Can you work these out from the model? Positions are in its coordinate system, mm. A direction names the side the tool comes from. Give positions to 0.01 mm unless a question says otherwise; leave off trailing zeros. Order: outer loops, then holes, each group sorted by start corner. A loop starts at its lowest first (then second) coordinate and runs counter-clockwise, first axis right, second up.
Item 1: If I drill on line 1 along X through (y, z) = (-21.55, 0); line 2 along X through (y, z) = (-23.2, 0); line 3 along X through (y, z) = (-21.65, 2.75), over which ranges is the centre line in solid material (lowest first)?
Item 2: I want a section at C-C, the plane z = -5.75. Write out the boundary of the cut face in (x, y), then the cut area to 3 significant figures.
Item 3: I want a section at A-A, the plane y = -21.15. Write out the boundary of the cut face in (x, z), then the cut area to 3 significant figures.
Item 4: Which directions (+Z, -Z, +X, -X, +Y, -Y) give clear straight access to the entire face, cutting with the end or side of a thin tool? Please do faces 5 (the cylindrical face through (-10.64, -21.87, 4.49)), 6 (the flat face through (-10.4, -22.03, -5.37)), 7 (the flat face through (-3, -23.5, -4)).
Item 5: I'm going to push flat-ended pins straight in: pin 1 Ø1.2 at (y, z) = (-22.5, 3) entering from +X; pin 2 Ø0.8 at (x, y) = (-1.5, -22.5) entering from -Z; pin 3 Ø6.5 at (x, z) = (1, 0) entering from +Y. Where does each tip first touch, or does it pass through?
Item 6: If we mould it in two halves opening along X, with no side actions, what happens to faces 1 (the flat face through (-2.724, -23.245, 0.537)), 2 (the cylindrical face through (-8.025, -22.028, 7.208)), 3 (the flat face through (4, -22, -4)), 4 (the flat face through (-7, -20, 7))? For each: +X half, -X half, draft (parallel to the pull), parting line (faces both ways), or undercut.
Item 7: I want a section at B-B, the plane x = 13. Write out the boundary of the cut face in (y, z).
Item 8: I want a section at D-D, the plane x = 2. Write out the boundary of the cut face in (y, z), then the cut area to 3 significant figures.
```python
from build123d import *

# Parameters (mm, degrees)
PAD096_DEPTH    = 4
SKETCH294_R     = 1.5
POCKET172_DEPTH = 6
SKETCH295_R     = 0.95
POCKET173_DEPTH = 1.5
SKETCH299_W     = 4.5
SKETCH299_H     = 8
POCKET175_DEPTH = 3
POCKET176_DEPTH = 5
POCKET177_DEPTH = 5
PAD107_DEPTH    = 2.5


with BuildPart() as part:
    # Sketch278 → Pad096 (new body)
    with BuildSketch(Plane.XZ.offset(24)):
        with BuildLine():
            Line((-17, -2.25), (-17, 2.25))
            ThreePointArc((-7, 7.25), (-12.5901699437, 5.9303398875), (-17, 2.25))
            Line((-7, 7.25), (0, 7.25))
            Line((0, 7.25), (0, -9.3))
            ThreePointArc((-3.9748544782, -8.4077661645), (-2.0368817676, -9.0742003871), (0, -9.3))
            Line((-3.9748544782, -8.4077661645), (-17, -2.25))
        make_face()
    pad096 = extrude(amount=-PAD096_DEPTH)

    # Sketch294 (on Face8 of Pad096) → Pocket172 (cut)
    with BuildSketch(Plane(origin=(0, -20, 0), x_dir=(1, 0, 0), z_dir=(0, 1, 0))):
        with Locations((-13, 0)):
            Circle(SKETCH294_R)
    pocket172 = extrude(amount=-POCKET172_DEPTH, mode=Mode.SUBTRACT)

    # Sketch295 (on Face5 of Pocket172) → Pocket173 (cut)
    with BuildSketch(Plane(origin=(0, -20, 0), x_dir=(1, 0, 0), z_dir=(0, 1, 0))):
        with BuildLine():
            Line((0, 9), (0, -9))
            ThreePointArc((-7.5, -4.9749371855), (-4.2559114964, -7.9301461106), (0, -9))
            Line((-7.5, -4.9749371855), (-7.5, 4.9749371855))
            ThreePointArc((0, 9), (-4.2559114964, 7.9301461106), (-7.5, 4.9749371855))
        make_face()
        with Locations((-6, 0)):
            Circle(SKETCH295_R, mode=Mode.SUBTRACT)
    pocket173 = extrude(amount=-POCKET173_DEPTH, mode=Mode.SUBTRACT)

    # Sketch299 (on Face5 of Pocket172) → Pocket175 (cut)
    with BuildSketch(Plane(origin=(0, -20, 0), x_dir=(1, 0, 0), z_dir=(0, 1, 0))):
        with Locations((-2.25, 0)):
            Rectangle(SKETCH299_W, SKETCH299_H)
    pocket175 = extrude(amount=-POCKET175_DEPTH, mode=Mode.SUBTRACT)

    # Mirrored012: Pad096, Pocket172, Pocket173, Pocket175 across Sketch278 V_Axis
    add(pad096.mirror(Plane(origin=(0, -24, 0), x_dir=(0, -1, 0), z_dir=(1, 0, 0))))
    add(pocket172.mirror(Plane(origin=(0, -24, 0), x_dir=(0, -1, 0), z_dir=(1, 0, 0))), mode=Mode.SUBTRACT)
    add(pocket173.mirror(Plane(origin=(0, -24, 0), x_dir=(0, -1, 0), z_dir=(1, 0, 0))), mode=Mode.SUBTRACT)
    add(pocket175.mirror(Plane(origin=(0, -24, 0), x_dir=(0, -1, 0), z_dir=(1, 0, 0))), mode=Mode.SUBTRACT)

    # Sketch300 → Pocket176 (cut)
    with BuildSketch(Plane.XZ.offset(24)):
        Polygon((-9, 0), (-13.5886114908, 6.5532163543), (-10.3120033137, 8.8475220997), (-5.7233918228, 2.2943057454), align=None)
    extrude(amount=-POCKET176_DEPTH, mode=Mode.SUBTRACT)

    # Sketch301 → Pocket177 (cut)
    with BuildSketch(Plane.XZ.offset(23.5)):
        with BuildLine():
            ThreePointArc((-3.5, -7.7459666924), (0, -8.5), (3.5, -7.7459666924))
            Line((3.5, -7.7459666924), (3.5, -3.7459666924))
            Line((3.5, -3.7459666924), (-6.7056942546, 3.2766081772))
            Line((-6.7056942546, 3.2766081772), (-9, 0))
            Line((-9, 0), (-3.5, -7.7459666924))
        make_face()
    extrude(amount=-POCKET177_DEPTH, mode=Mode.SUBTRACT)

    # Sketch302 (on Face13 of Pocket177) → Pad107 (join)
    with BuildSketch(Plane(origin=(-6.039090645, 0, -4.2286167935), x_dir=(-0.5735764364, 0, 0.8191520443), z_dir=(0.8191520443, 0, 0.5735764364))):
        with BuildLine():
            Line((12, 20), (12, 23))
            ThreePointArc((7.4, 21.5), (9.8191940807, 21.8844714859), (12, 23))
            Line((7.4, 21.5), (7.4, 20))
            Line((7.4, 20), (12, 20))
        make_face()
    extrude(amount=PAD107_DEPTH)


solid = part.part
```
Results list:
1. line 1: x = -17 to -14.5, -11.5 to -9, 4.5 to 11.5, 14.5 to 17
1. line 2: x = -17 to -14.5, -11.5 to -9, -1.94 to 11.5, 14.5 to 17
1. line 3: x = -16.6 to -10.93, -5.94 to -4.5, 4.5 to 16.6
2. outline: (-9.6, -24) - (9.6, -24) - (9.6, -20) - (6.92, -20) - (6.92, -21.5) - (3.5, -21.5) - (3.5, -23.5) - (-4.92, -23.5) - (-4.92, -21.5) - (-6.92, -21.5) - (-6.92, -20) - (-9.6, -20) - close
2. area: 39.2 mm2
3. outline: (-17, -2.25) - (-3.97, -8.41) arc R9.3 ccw to (3.97, -8.41) - (17, -2.25) - (17, 2.25) arc R12.5 ccw to (7, 7.25) - (5.33, 7.25) arc R9 cw to (7.5, 4.97) - (7.5, -4.97) arc R9 cw to (-7.5, -4.97) - (-7.5, -2.11) - (-9, 0) - (-10.28, 1.83) - (-8.24, 3.27) - (-10.87, 7.04) - (-12.92, 5.6) - (-13, 5.71) arc R12.5 ccw to (-17, 2.25) - close; (-9.07, 7.08) - (-7.5, 4.83) - (-7.5, 4.97) arc R9 cw to (-5.33, 7.25) - (-7, 7.25) arc R12.5 ccw to start; circle Ø1.9 at (6, 0); hole circle Ø3 at (-13, 0); hole circle Ø3 at (13, 0)
3. area: 180 mm2
4. face 5: -Y
4. face 6: -Z, -X, +Y, -Y
4. face 7: +Y
5. pin 1: stops at x = 16.89
5. pin 2: stops at z = -9.23
5. pin 3: stops at y = -23
6. face 1: undercut
6. face 2: -X half
6. face 3: undercut
6. face 4: draft
7. outline: (-24, -4.14) - (-20, -4.14) - (-20, -1.5) - (-24, -1.5) - close; (-24, 1.5) - (-20, 1.5) - (-20, 5.72) - (-24, 5.72) - close
8. outline: (-24, -9.08) - (-20, -9.08) - (-20, -8.77) - (-21.5, -8.77) - (-21.5, -8.26) - (-23.5, -8.26) - (-23.5, -2.71) - (-23, -2.71) - (-23, 4) - (-21.5, 4) - (-21.5, 7.25) - (-24, 7.25) - close
8. area: 20.1 mm2
